Study the drawing (mm; zero at the part's minimum x, y, z) and answer. A direction names the side the tool comes from. Coordinates: 2 decimals unless noted, no trailing zeros. Loops run counter-clockwise (first coordinate to the right, second up) from the corner with the lowest first, then second, coordinate; pieces in that order, holes last. Notation, with made-up numbers: (-21.5, 49.25) - (3.5, 49.25) arc R16 ccw to (3.5, 54.25) - close; hole circle Ø2 at (-11, 17). An arc over 180 degrees is marked (long way). Use CSV: the item, a comma, the result in double quotes.
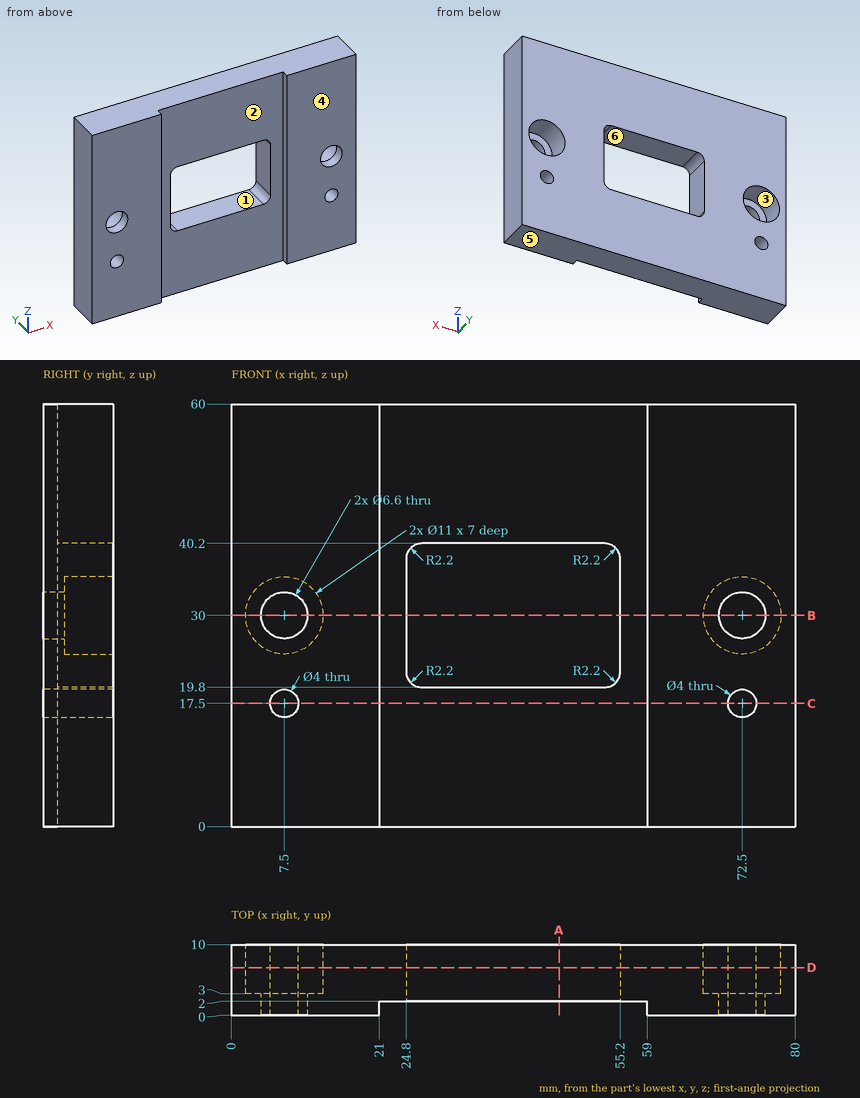
Q1. The part is cut by section A-A on x = 46.5. Determine the outline of the cut face in (y, z), and give its area (3 significant figures).
Reported:
outline,"(2, 0) - (10, 0) - (10, 19.8) - (2, 19.8) - close; (2, 40.2) - (10, 40.2) - (10, 60) - (2, 60) - close"
area,"317 mm²"
Q2. A tool of negligible diameter and unlimited length cuts with its end or side. For the marked faces 1, 2 and 3, from which of +Z, -Z, +X, -X, +Y, -Y can it reach the whole face along a straight path? Write none if from no direction.
Reported:
face 1,"+Y, -Y"
face 2,"+Z, -Z, -Y"
face 3,"+Y"
Q3. For a pull along Z with two mould halves and no side action, classify the marked faces 4, 5 and 6 as +Z half, -Z half, draft (parallel to the pull), parting line (faces both ways), or undercut.
Reported:
face 4,"draft"
face 5,"-Z half"
face 6,"undercut"
Q4. Find the intervals of material crossed by probe 1 along X at (y, z) = (1.25, 30); probe 2 along X at (y, z) = (1.5, 12.5); probe 3 along X at (y, z) = (7.5, 17.5), in increasing order. Write a range as [from, to].
Reported:
probe 1,"x = [0, 4.2], [10.8, 21], [59, 69.2], [75.8, 80]"
probe 2,"x = [0, 21], [59, 80]"
probe 3,"x = [0, 5.5], [9.5, 70.5], [74.5, 80]"
Q5. Given P1, Ø3, axis at x = 10, y = 7, coming from the -Z side; P2, Ø3.5, axis at x = 75, z = 30.5, coming from the +Y side, each flat-ended and moving along its own axis, determine where each tip first touches the part or whether it passes through.
Reported:
P1,"stops at z = 0"
P2,"stops at y = 3"
Q6. The part is cut by section C-C on z = 17.5. Determine the outline of the cut face in (x, y), and give its area (3 significant figures).
Reported:
outline,"(0, 0) - (5.5, 0) - (5.5, 10) - (0, 10) - close; (9.5, 0) - (21, 0) - (21, 2) - (59, 2) - (59, 0) - (70.5, 0) - (70.5, 10) - (9.5, 10) - close; (74.5, 0) - (80, 0) - (80, 10) - (74.5, 10) - close"
area,"644 mm²"
Q7. The part is cut by section D-D on y = 6.75. Determine the outline of the cut face in (x, z), and give its area (3 significant figures).
Reported:
outline,"(0, 0) - (80, 0) - (80, 60) - (0, 60) - close; hole circle Ø11 at (7.5, 30); hole circle Ø4 at (7.5, 17.5); hole (24.8, 22) arc R2.2 ccw to (27, 19.8) - (53, 19.8) arc R2.2 ccw to (55.2, 22) - (55.2, 38) arc R2.2 ccw to (53, 40.2) - (27, 40.2) arc R2.2 ccw to (24.8, 38) - close; hole circle Ø11 at (72.5, 30); hole circle Ø4 at (72.5, 17.5)"
area,"3,970 mm²"
Q8. The part is cut by section B-B on z = 30. Determine the outline of the cut face in (x, y), and give its area (3 significant figures).
Reported:
outline,"(0, 0) - (4.2, 0) - (4.2, 3) - (2, 3) - (2, 10) - (0, 10) - close; (10.8, 0) - (21, 0) - (21, 2) - (24.8, 2) - (24.8, 10) - (13, 10) - (13, 3) - (10.8, 3) - close; (55.2, 2) - (59, 2) - (59, 0) - (69.2, 0) - (69.2, 3) - (67, 3) - (67, 10) - (55.2, 10) - close; (75.8, 0) - (80, 0) - (80, 10) - (78, 10) - (78, 3) - (75.8, 3) - close"
area,"287 mm²"
